```python
from build123d import *

# Parameters (mm, degrees)
EXTRUDE_1_DEPTH     = 10
CUT_EXTRUDE_1_REACH = 32
SKETCH_3_R          = 1.75


with BuildPart() as part:
    # Эскиз2 → Бобышка-Вытянуть1 (new body)
    with BuildSketch(Plane.XY):
        Polygon((0, 0), (0, 20), (1.5, 20), (1.5, 1.5), (20, 1.5), (20, 0), align=None)
    extrude(amount=EXTRUDE_1_DEPTH)

    # Эскиз3 → Вырез-Вытянуть1 (cut, up to next)
    with BuildSketch(Plane.XZ, mode=Mode.PRIVATE) as cut_extrude_1_sk1:
        with Locations((10, 5)):
            Circle(SKETCH_3_R)
    cut_extrude_1_tool1 = extrude(cut_extrude_1_sk1.sketch, amount=-CUT_EXTRUDE_1_REACH, mode=Mode.PRIVATE) & part.part
    cut_extrude_1 = cut_extrude_1_tool1.solids().sort_by_distance((10, 0, 5))[0]
    add(cut_extrude_1, mode=Mode.SUBTRACT)

    # Зеркальное отражение1: Вырез-Вытянуть1 across plane
    add(cut_extrude_1.mirror(Plane(origin=(0, 0, 0), x_dir=(0, 0, 1), z_dir=(-0.7071067811865471, 0.7071067811865479, 0))), mode=Mode.SUBTRACT)


solid = part.part
```
Geometry check sheet. Reference: the model listing, model coordinates, mm. A direction names the side the tool comes from. Coordinates: 2 decimals unless noted, no trailing zeros. Order: outer loops, then holes, each group sorted by start corner. A loop starts at its lowest first (then second) coordinate and runs counter-clockwise, first axis right, second up. Notation, with made-up numbers: (-6.75, -36) - (39.25, -36) arc R13 cw to (39.25, -16) - close; hole circle Ø11 at (74, 13). An arc over 180 degrees is marked (long way). Answer as a JSON object with one key per item and string values. Group by question number.
Item 1: Depth check by flat-ended pin: pin 1 Ø4 at (x, z) = (6, 6.5) entering from +Y. Enter the tip coordinate at first touch or a pass-through.
Item 2: Tool access check on faces 4 (the face through (1, 20, 5)), 5 (the face through (13, 1.5, 5)). Record the directions out of +Z, -Z, +X, -X, +Y, -Y that give a thin tool (end or side, any length) a straight path to the whole face; none if there is none.
Item 3: Sectioned sample at B-B, the plane z = 5. Record the cut outline in (x, y), and give its area (4 significant figures).
Item 4: Sectioned sample at D-D, the plane z = 1.25. Record the cut outline in (x, y), and give its area (4 significant figures).
Item 5: Draft check along Z on faces 1 (the face through (12, 0, 5)), 2 (the face through (6, 1, 10)), 3 (the face through (0.74, 11.617, 4.33)). Enter one of: +Z half, -Z half, draft (parallel to the pull), parting line (faces both ways), or undercut.
Item 6: Sectioned sample at A-A, the plane y = 10. Record the cut outline in (x, z).
Item 7: Scan lines: probe 1 along Z at (x, y) = (10, 0.45); probe 2 along X at (y, z) = (15.75, 3.25). Record each from-to range of solid material in increasing order.
Resolved:
{
 "1": {"pin 1": "y = 1.5"},
 "2": {"face 4": "+Z, -Z, +X, -X, +Y", "face 5": "+Z, -Z, +X, +Y"},
 "3": {"outline": "(0, 0) - (8.25, 0) - (8.25, 1.5) - (1.5, 1.5) - (1.5, 8.25) - (0, 8.25) - close; (0, 11.75) - (1.5, 11.75) - (1.5, 20) - (0, 20) - close; (11.75, 0) - (20, 0) - (20, 1.5) - (11.75, 1.5) - close", "area": "47.25 mm^2"},
 "4": {"outline": "(0, 0) - (20, 0) - (20, 1.5) - (1.5, 1.5) - (1.5, 20) - (0, 20) - close", "area": "57.75 mm^2"},
 "5": {"face 1": "draft", "face 2": "+Z half", "face 3": "undercut"},
 "6": {"outline": "(0, 0) - (1.5, 0) - (1.5, 3.25) - (0, 3.25) - close; (0, 6.75) - (1.5, 6.75) - (1.5, 10) - (0, 10) - close"},
 "7": {"probe 1": "0 to 3.25, 6.75 to 10", "probe 2": "0 to 1.5"}
}
